Autodesk Inventor part; units mm, degrees
ref_plane "Work Plane1" through (0, 0, 26) normal (0, 0, 1) x (1, 0, 0)
ref_plane "Work Plane2" through (0, 0, 61) normal (0, 0, 1) x (1, 0, 0)
ref_plane "YZ Plane" through (0, 0, 0) normal (1, 0, 0) x (0, 1, 0)
sketch "Sketch1" plane through (0, 0, 0) normal (0, 0, 1) x (1, 0, 0)
  line L0 (0, 0) -> (80, 0)
  line L1 (80, 0) -> (80, 50)
  line L2 (80, 50) -> (0, 50)
  line L3 (0, 50) -> (0, 0)
  dimension "d0" = 80
  dimension "d1" = 50
extrude "Extrusion1" add sketch "Sketch1" along normal blind 6
sketch "Sketch2" plane through (0, 0, 6) normal (0, 0, 1) x (1, 0, 0)
  line L0 (80, 50) -> (0, 50)
  line L1 (0, 50) -> (0, 0)
  arc A0 (60.1556, 0) -> (19.8444, 0) centre (40, 10) ccw
  line L2 (19.8444, 0) -> (60.1556, 0)
  dimension "d11" = 45
  dimension "d12" = 40
  dimension "d13" = 40
  dimension "d14" = 10
extrude "Extrusion2" add sketch "Sketch2" along normal blind 75
sketch "Sketch8" plane through (0, 0, 81) normal (0, 0, 1) x (1, 0, 0)
  arc A0 (60.1556, 0) -> (19.8444, 0) centre (40, 10) ccw
  line L0 (19.8444, 0) -> (60.1556, 0)
  arc A1 (63.4574, 0) -> (16.5426, 0) centre (40, 10) ccw
  line L1 (19.8444, 0) -> (16.5426, 0)
  line L2 (60.1556, 0) -> (63.4574, 0)
  point P0 (0, 0)
  dimension "d30" = 51
extrude "Extrusion7" add sketch "Sketch8" along normal blind 4
sketch "Sketch9" plane through (0, 0, 0) normal (0, 0, -1) x (-1, 0, 0)
  line L0 (0, 0) -> (-80, 0)
  line L1 (-80, 0) -> (-80, 50)
  point P0 (-72.5, 42.5)
  point P1 (-72.5, 7.5)
  point P2 (-7.5, 42.5)
  point P3 (-7.5, 7.5)
  dimension "d33" = 65
  dimension "d34" = 35
  dimension "d35" = 7.5
  dimension "d36" = 7.5
hole "Hole1" at (72.5, 42.5, 0) at (72.5, 7.5, 0) at (7.5, 42.5, 0) at (7.5, 7.5, 0) direction (0, 0, 1) diameter 4.5 end through all
sketch "Sketch10" plane through (0, 0, 6) normal (0, 0, 1) x (1, 0, 0)
  circle A0 centre (7.5, 42.5) radius 2.25
  circle A1 centre (72.5, 42.5) radius 2.25
  circle A2 centre (72.5, 7.5) radius 2.25
  circle A3 centre (7.5, 7.5) radius 2.25
  line L0 (11.7724, 42.5) -> (9.6362, 38.8)
  line L1 (9.6362, 38.8) -> (5.3638, 38.8)
  line L2 (5.3638, 38.8) -> (3.2276, 42.5)
  line L3 (3.2276, 42.5) -> (5.3638, 46.2)
  line L4 (5.3638, 46.2) -> (9.6362, 46.2)
  line L5 (9.6362, 46.2) -> (11.7724, 42.5)
  line L6 (11.7724, 7.5) -> (9.6362, 3.8)
  line L7 (9.6362, 3.8) -> (5.3638, 3.8)
  line L8 (5.3638, 3.8) -> (3.2276, 7.5)
  line L9 (3.2276, 7.5) -> (5.3638, 11.2)
  line L10 (5.3638, 11.2) -> (9.6362, 11.2)
  line L11 (9.6362, 11.2) -> (11.7724, 7.5)
  line L12 (76.7724, 7.5) -> (74.6362, 3.8)
  line L13 (74.6362, 3.8) -> (70.3638, 3.8)
  line L14 (70.3638, 3.8) -> (68.2276, 7.5)
  line L15 (68.2276, 7.5) -> (70.3638, 11.2)
  line L16 (70.3638, 11.2) -> (74.6362, 11.2)
  line L17 (74.6362, 11.2) -> (76.7724, 7.5)
  line L18 (76.7724, 42.5) -> (74.6362, 38.8)
  line L19 (74.6362, 38.8) -> (70.3638, 38.8)
  line L20 (70.3638, 38.8) -> (68.2276, 42.5)
  line L21 (68.2276, 42.5) -> (70.3638, 46.2)
  line L22 (70.3638, 46.2) -> (74.6362, 46.2)
  line L23 (74.6362, 46.2) -> (76.7724, 42.5)
  dimension "d44" = 7.4
extrude "Extrusion8" cut sketch "Sketch10" against normal blind 3.5
sketch "Sketch4" plane through (0, 0, 26) normal (0, 0, 1) x (1, 0, 0)
  arc A0 (62.9129, 0) -> (17.0871, 0) centre (40, 10) ccw
  line L0 (17.0871, 0) -> (62.9129, 0)
  circle A1 centre (40, 24.5) radius 11 construction
  arc A2 (28, 24.5) -> (52, 24.5) centre (40, 24.5) ccw
  line L1 (28, 24.5) -> (28, 31.9317)
  line L2 (52, 24.5) -> (52, 31.9317)
  arc A3 (62.9129, 0) -> (17.0871, 0) centre (40, 10) ccw
  point P0 (0, 0)
  dimension "d15" = 22
  dimension "d16" = 14.5
  dimension "d17" = 24
sketch "Sketch5" plane through (0, 0, 61) normal (0, 0, 1) x (1, 0, 0)
  arc A0 (62.9129, 0) -> (17.0871, 0) centre (40, 10) ccw
  line L0 (17.0871, 0) -> (62.9129, 0)
  arc A1 (28, 24.5) -> (52, 24.5) centre (40, 24.5) ccw
  line L1 (52, 31.9317) -> (52, 24.5)
  arc A2 (52, 31.9317) -> (28, 31.9317) centre (40, 10) ccw
  line L2 (28, 24.5) -> (28, 31.9317)
  point P0 (0, 0)
sketch "Sketch6" plane through (0, 0, 26) normal (0, 0, 1) x (1, 0, 0)
  arc A0 (28, 24.5) -> (52, 24.5) centre (40, 24.5) ccw
  line L0 (52, 31.9317) -> (52, 24.5)
  arc A1 (52, 31.9317) -> (28, 31.9317) centre (40, 10) ccw
  line L1 (28, 24.5) -> (28, 31.9317)
  arc A2 (35.75, 24.5) -> (44.25, 24.5) centre (40, 24.5) ccw
  line L2 (35.75, 26.9) -> (35.75, 34.6361)
  arc A3 (52, 31.9317) -> (28, 31.9317) centre (40, 10) ccw
  line L3 (44.25, 26.9) -> (44.25, 34.6361)
  arc A4 (35.75, 24.5) -> (35.75, 26.9) centre (34.15, 25.7) ccw
  arc A5 (44.25, 26.9) -> (44.25, 24.5) centre (45.85, 25.7) ccw
  point P0 (0, 0)
  dimension "d23" = 8.5
  dimension "d24" = 2
  dimension "d25" = 1.6
sketch "Sketch7" plane through (0, 0, 61) normal (0, 0, 1) x (1, 0, 0)
  arc A0 (35.75, 24.5) -> (44.25, 24.5) centre (40, 24.5) ccw
  arc A1 (44.25, 26.9) -> (44.25, 24.5) centre (45.85, 25.7) ccw
  line L0 (44.25, 34.6361) -> (44.25, 26.9)
  arc A2 (44.25, 34.6361) -> (35.75, 34.6361) centre (40, 10) ccw
  line L1 (35.75, 26.9) -> (35.75, 34.6361)
  arc A3 (35.75, 24.5) -> (35.75, 26.9) centre (34.15, 25.7) ccw
  point P0 (0, 0)
properties part number "SpoolHolderSingle" material "ABS Plastic"
The listing builds one solid part. Answer for the finished solid, in the listing's coordinates (mm). A direction names the side the tool comes from. Round coordinates to 2 decimals unless told otherwise and drop trailing zeros. Order: outer loops, then holes, each group sorted by start corner. A loop starts at its lowest first (then second) coordinate and runs counter-clockwise, first axis right, second up. Notation, with made-up numbers: (27, 4.5) - (73, 4.5) arc R30 cw to (73, 39.5) - close; hole circle Ø7 at (76.5, 70). An arc over 180 degrees is marked (long way). Write item = value, one per line. Start each with the question number.
1) Given pin 1 (12 mm diameter, centred on x = 53, z = 26, fed in from -Y); pin 2 (8 mm diameter, centred on x = 71, y = 8.5, fed in from +Z); pin 3 (5 mm diameter, centred on x = 7.5, y = 7.5, fed in from +Z); pin 4 (2 mm diameter, centred on x = 61, z = 41.5, fed in from +Y), each flat-ended and moving along its own axis, determine where each tip first touches the part or whether it passes through.
2) Section B-B, the plane x = 40 is taken. Write down the section's boundary in (y, z).
3) For faces 1 (the flat face through (73, 3.8, 4)), 2 (the cylindrical face through (74.696, 7.012, 1.268)), determine the directions among +Z, -Z, +X, -X, +Y, -Y from which every point of the face is accessible in a straight line to the end or side of a thin tool.
4) Straight lines are drawn through the part: L1, parallel to Y at x = 7.5, z = 1.35; L2, parallel to X at y = 42, z = 1; L3, parallel to Z at x = 39, y = 35. For each, find the intervals that lie inside material, in ascending order.
5) For a pull along X with two mould halves and no side action, classify faces 3 (the flat face through (7, 46.2, 4)), 4 (the flat face through (39, 0, 42)), 5 (the flat face through (4.311, 5.624, 4.274)), 6 (the cylindrical face through (39.3, 35.49, 82.97)) as released by +X, released by -X, zero draft, split by the parting line, or undercut.
6) Section D-D, the plane y = 30 is taken. Write down the section's boundary in (x, z), plus the area to 3 significant figures.
7) Section C-C, the plane y = 19 is taken. Write down the section's boundary in (x, z), plus the area to 3 significant figures.
8) Section A-A, the plane x = 7.5 is taken. Write down the section's boundary in (y, z).
Results list:
q1.pin_1 = 0
q1.pin_2 = 6
q1.pin_3 = 2.5
q1.pin_4 = 20.31
q2.outline = (0, 0) - (50, 0) - (50, 6) - (32.5, 6) - (32.5, 81) - (35.5, 81) - (35.5, 85) - (0, 85) - close
q3.face_1 = +Z
q3.face_2 = +Z, -Z
q4.L1 = 0 to 5.25, 9.75 to 40.25, 44.75 to 50
q4.L2 = 0 to 5.31, 9.69 to 70.31, 74.69 to 80
q4.L3 = 0 to 6, 81 to 85
q5.face_3 = undercut
q5.face_4 = zero draft
q5.face_5 = undercut
q5.face_6 = split by the parting line
q6.outline = (0, 0) - (80, 0) - (80, 6) - (50.31, 6) - (50.31, 81) - (55.82, 81) - (55.82, 85) - (24.18, 85) - (24.18, 81) - (29.69, 81) - (29.69, 6) - (0, 6) - close
q6.area = 2,150 mm^2
q7.outline = (0, 0) - (80, 0) - (80, 6) - (60.62, 6) - (60.62, 81) - (63.86, 81) - (63.86, 85) - (16.14, 85) - (16.14, 81) - (19.38, 81) - (19.38, 6) - (0, 6) - close
q7.area = 3,760 mm^2
q8.outline = (0, 0) - (5.25, 0) - (5.25, 2.5) - (3.8, 2.5) - (3.8, 6) - (0, 6) - close; (9.75, 0) - (40.25, 0) - (40.25, 2.5) - (38.8, 2.5) - (38.8, 6) - (11.2, 6) - (11.2, 2.5) - (9.75, 2.5) - close; (44.75, 0) - (50, 0) - (50, 6) - (46.2, 6) - (46.2, 2.5) - (44.75, 2.5) - close
